from build123d import *

# Parameters (mm, degrees)
F3_R     = 2.032
F4_DEPTH = 9.526
F5_DEPTH = 9.526
F6_DEPTH = 7.2644
F7_R     = 5.08


with BuildPart() as f2:
    # F1 (on Front) → F2 (revolve)
    with BuildSketch(Plane.XZ):
        with BuildLine():
            Line((45.953082, -2.622399), (45.953082, 0))
            Line((45.953082, 0), (0, 0))
            Line((0, 0), (0, -9.525))
            Line((0, -9.525), (45.953082, -9.525))
            Line((45.953082, -9.525), (45.953082, -7.194399))
            ThreePointArc((45.953082, -7.194399), (43.667082, -4.908399), (45.953082, -2.622399))
        make_face()
    revolve(axis=Axis((0, 0, -4.7625), (0, 0, -1)))

    # F3 (on face) → F4 (cut, through all)
    with BuildSketch(Plane(origin=(0, 0, -9.525), x_dir=(1, 0, 0), z_dir=(0, 0, -1))):
        Circle(F3_R)
    extrude(amount=-F4_DEPTH, mode=Mode.SUBTRACT)

    # F0 (on Top) → F5 (cut, through all)
    with BuildSketch(Plane.XY):
        with BuildLine():
            Line((-3.812821, 8.537283), (32.424712, 24.721265))
            ThreePointArc((32.424712, 24.721265), (9.907948, 39.551681), (-16.941164, 37.087731))
            Line((-16.941164, 37.087731), (-3.812821, 8.537283))
        make_face()
        with BuildLine():
            Line((-7.404719, 5.709023), (-20.882838, 35.020136))
            ThreePointArc((-20.882838, 35.020136), (-32.656298, 24.414526), (-39.497569, 10.121508))
            Line((-39.497569, 10.121508), (-9.307396, -0.891727))
            ThreePointArc((-9.307396, -0.891727), (-9.349033, -0.135558), (-9.329338, 0.6215))
            ThreePointArc((-9.329338, 0.6215), (-8.745163, 3.308311), (-7.404719, 5.709023))
        make_face()
        with BuildLine():
            ThreePointArc((-40.372143, 5.709023), (-37.814361, -15.250474), (-25.115689, -32.120165))
            Line((-25.115689, -32.120165), (-2.147453, -9.100069))
            ThreePointArc((-2.147453, -9.100069), (-4.557398, -8.164124), (-6.618911, -6.604))
            Line((-6.618911, -6.604), (-40.372143, 5.709023))
        make_face()
        with BuildLine():
            ThreePointArc((-21.412568, -34.698772), (7.22509, -40.128555), (32.170471, -25.051221))
            Line((32.170471, -25.051221), (9.001197, -2.530069))
            ThreePointArc((9.001197, -2.530069), (8.071318, -4.719812), (6.618911, -6.604))
            Line((6.618911, -6.604), (-21.412568, -34.698772))
        make_face()
        with BuildLine():
            ThreePointArc((34.738316, -21.348355), (39.235928, -11.092558), (40.773801, 0))
            ThreePointArc((40.773801, 0), (39.293229, 10.887838), (34.959038, 20.98496))
            Line((34.959038, 20.98496), (5.268002, 7.724698))
            ThreePointArc((5.268002, 7.724698), (6.961236, 6.242114), (8.251151, 4.397876))
            Line((8.251151, 4.397876), (34.738316, -21.348355))
        make_face()
    extrude(amount=-F5_DEPTH, mode=Mode.SUBTRACT)

    # F0 (on Top) → F6 (cut)
    with BuildSketch(Plane.XY):
        Polygon((-3.812821, 6.604), (-7.625642, 0), (-3.812821, -6.604), (3.812821, -6.604), (7.625642, 0), (3.812821, 6.604), align=None)
    extrude(amount=-F6_DEPTH, mode=Mode.SUBTRACT)

    # F7
    f7_edges = [f2.edges().sort_by_distance(p)[0] for p in [
        (34.959038, 20.98496, -4.7625),
        (32.424712, 24.721265, -4.7625),
        (-16.941164, 37.087731, -4.7625),
        (-20.882838, 35.020136, -4.7625),
        (-39.497569, 10.121508, -4.7625),
        (-40.372143, 5.709023, -4.7625),
        (-21.412568, -34.698772, -4.7625),
        (-25.115689, -32.120165, -4.7625),
        (32.170471, -25.051221, -4.7625),
        (34.738316, -21.348355, -4.7625),
    ]]
    fillet(f7_edges, radius=F7_R)


solid = f2.part
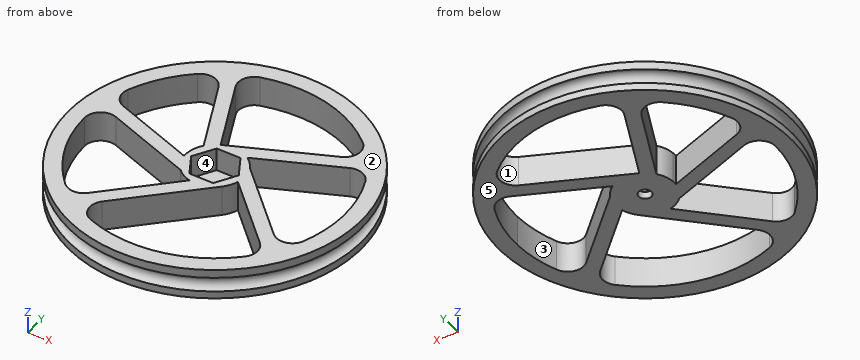
Verification items for the finished model (mm, model axes). Face numbers are marked on the shaded views. A direction names the side the tool comes from. Give positions to 0.01 mm unless a question says otherwise; leave off trailing zeros. Loops run counter-clockwise (first coordinate to the right, second up) from the corner with the lowest first, then second, coordinate; pieces in that order, holes last.
1) Depth check by flat-ended pin: pin 1 Ø5 at (y, z) = (34, -5) entering from +X; pin 2 Ø5 at (x, z) = (17, -5) entering from -Y; pin 3 Ø1.5 at (y, z) = (-36, -6) entering from -X. Enter the tip coordinate at first touch or a pass-through.
2) Set-up check for the marked faces 3, 4 and 5: record each of +Z, -Z, +X, -X, +Y, -Y from which the full face is reachable in a straight line by a thin tool's end or side.
3) Thickness scan on line 1 along Y through (x, z) = (-24, -2.25); line 2 along Y through (x, z) = (-7.5, -2); line 3 along Y through (x, z) = (0, -7.75). Record the ranges inside material, lowest first.
4) Draft check along X on the marked faces 1 and 2. Enter one of: pulls with the +X half, pulls with the -X half, needs draft (parallel to the pull), parting line crosses it, or undercut.
5) Sectioned sample at A-A, the plane x = 0. Enter the section's corners in (y, z) (3 decimals).
6) Sectioned sample at B-B, the plane y = 27.5. Count the separate pieces of the cut face and the enclosed holes in it, then the cut area to 3 significant figures.
Answers:
1. pin 1: stops at x = 32.18
1. pin 2: stops at y = -43.15
1. pin 3: stops at x = -26.63
2. face 3: +Z, -Z
2. face 4: +Z
2. face 5: -Z, +X, -X, +Y, -Y
3. line 1: y = -39.19 to -30.05, -0.26 to 4.47, 32.31 to 39.19
3. line 2: y = -45.34 to -40.08, -20.75 to -14.46, -6.28 to -0.22, 0.22 to 5.58, 5.92 to 16.56, 40.08 to 45.34
3. line 3: y = -45.95 to -40.77, -13.24 to -2.03, 2.03 to 10.24, 40.77 to 45.95
4. face 1: undercut
4. face 2: needs draft
5. outline: (-45.953, -9.525) - (-40.774, -9.525) - (-40.774, 0) - (-45.953, 0) - (-45.953, -2.622) arc R2.286 cw to (-45.953, -7.194) - close; (-13.238, -9.525) - (-2.032, -9.525) - (-2.032, -7.264) - (-6.604, -7.264) - (-6.604, 0) - (-13.238, 0) - close; (2.032, -9.525) - (10.24, -9.525) - (10.24, 0) - (6.604, 0) - (6.604, -7.264) - (2.032, -7.264) - close; (40.774, -9.525) - (45.953, -9.525) - (45.953, -7.194) arc R2.286 cw to (45.953, -2.622) - (45.953, 0) - (40.774, 0) - close
6. separate pieces: 3
6. enclosed holes: 0
6. area: 165 mm2
